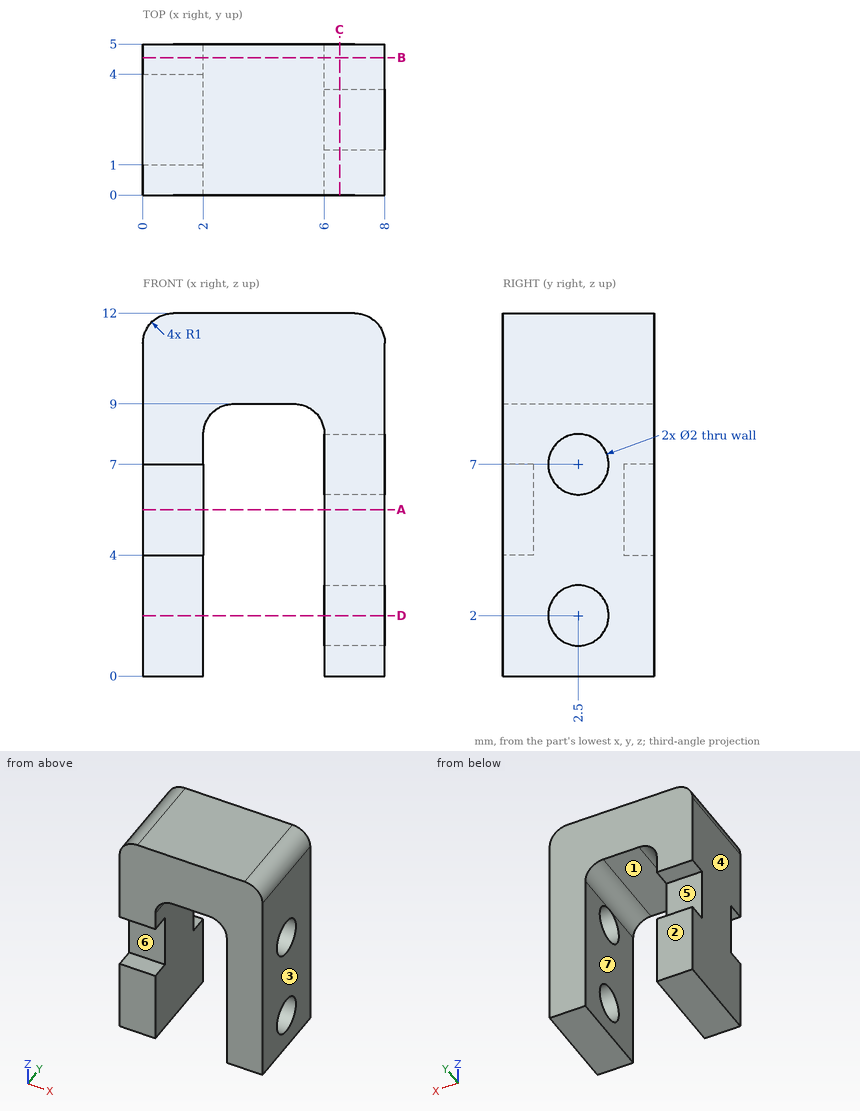
Part print with two shaded views. Sizes in mm from the minimum x, y, z corner. A direction names the side the tool comes from. Give positions to 0.01 mm unless a question says otherwise; leave off trailing zeros. Order: outer loops, then holes, each group sorted by start corner. A loop starts at its lowest first (then second) coordinate and runs counter-clockwise, first axis right, second up.
(1) Saw through at C-C, the plane x = 6.5. Give the cut face in (y, z), then the cut area to 3 significant figures.
(2) Saw through at B-B, the plane y = 4.55. Give the cut face in (x, z).
(3) Saw through at A-A, the plane z = 5.5. Give the cut face in (x, y), then the cut area to 3 significant figures.
(4) Saw through at D-D, the plane z = 2. Give the cut face in (x, y), then the cut area to 3 significant figures.
(5) Tool access for the marked faces 5, 6 and 7: list every direction of +Z, -Z, +X, -X, +Y, -Y with a clear straight run to the whole face (end or side of a thin tool).
(6) Flat gauge pins, fed straight in: pin 1 (1.2 mm diameter, centred on y = 2.5, z = 7, fed in from +X); pin 2 (2 mm diameter, centred on x = 3.5, y = 3.5, fed in from -Z); pin 3 (0.6 mm diameter, centred on x = 1.5, z = 5.5, fed in from +Y). Where does each tip first touch, or does it go through?
(7) Drill centre lines: L1, parallel to X at y = 0.8, z = 1; L2, parallel to Y at x = 6.8, z = 2; L3, parallel to Z at x = 4, y = 3.4. Where is each one in solid material? Low to high.
(8) Mould opens along X. For the marked faces 1, 2, 3 and 4 say: released by +X, released by -X, zero draft, split by the parting line, or undercut.
Results found:
1. outline: (0, 0) - (5, 0) - (5, 12) - (0, 12) - close; hole circle Ø2 at (2.5, 2); hole circle Ø2 at (2.5, 7)
1. area: 53.7 mm2
2. outline: (0, 0) - (2, 0) - (2, 4) - (0, 4) - close; (0, 7) - (2, 7) - (2, 8) arc R1 cw to (3, 9) - (5, 9) arc R1 cw to (6, 8) - (6, 0) - (8, 0) - (8, 11) arc R1 ccw to (7, 12) - (1, 12) arc R1 ccw to (0, 11) - close
3. outline: (0, 1) - (2, 1) - (2, 4) - (0, 4) - close; (6, 0) - (8, 0) - (8, 5) - (6, 5) - close
3. area: 16.0 mm2
4. outline: (0, 0) - (2, 0) - (2, 5) - (0, 5) - close; (6, 0) - (8, 0) - (8, 1.5) - (6, 1.5) - close; (6, 3.5) - (8, 3.5) - (8, 5) - (6, 5) - close
4. area: 16.0 mm2
5. face 5: -X, +Y
5. face 6: -X, -Y
5. face 7: -Z, +Y, -Y
6. pin 1: stops at x = 2
6. pin 2: stops at z = 8.87
6. pin 3: stops at y = 4
7. L1: x = 0 to 2, 6 to 8
7. L2: y = 0 to 1.5, 3.5 to 5
7. L3: z = 9 to 12
8. face 1: undercut
8. face 2: zero draft
8. face 3: released by +X
8. face 4: released by -X
